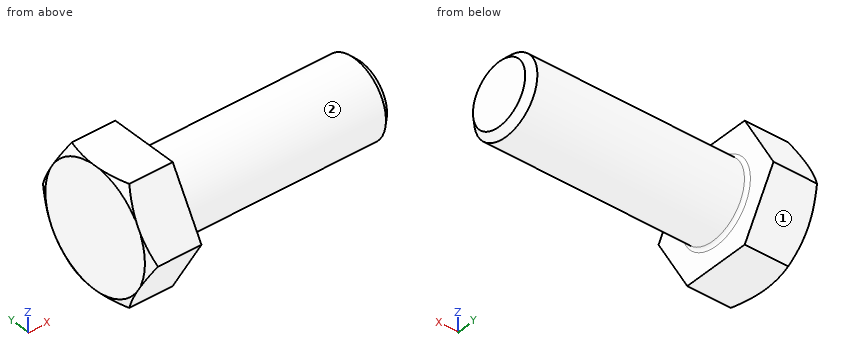
Autodesk Inventor part; units mm, degrees
ref_plane "Work Plane1" through (1.525, 0, 0) normal (0, 0, 1) x (1, 0, 0)
ref_plane "YZ Plane" through (0, 0, 0) normal (1, 0, 0) x (0, 1, 0)
ref_plane "XZ Plane" through (0, 0, 0) normal (0, 1, 0) x (-1, 0, 0)
sketch "Sketch1" plane through (0, 0, 0) normal (0, 0, 1) x (1, 0, 0)
  line L0 (0, 3.5) -> (20, 3.5)
  line L1 (20, 3.5) -> (20, 0)
  line L2 (20, 0) -> (0, 0)
  line L3 (-4, 0) -> (24, 0)
  line L4 (0, -0.7) -> (0, 4.2)
  line L5 (0, 3.5) -> (0, 0)
  dimension "d2" = 7
  dimension "d59" = 20
revolve "Body" add sketch "Sketch1" angle 360 about axis through (20, 0, 0) along (-1, 0, 0)
sketch "Sketch2" plane through (0, 0, 0) normal (-1, 0, 0) x (0, 0, 1)
  line L0 (0, 6.3509) -> (5.5, 3.1754)
  line L1 (5.5, 3.1754) -> (5.5, -3.1754)
  line L2 (5.5, -3.1754) -> (0, -6.3509)
  line L3 (0, -6.3509) -> (-5.5, -3.1754)
  line L4 (-5.5, -3.1754) -> (-5.5, 3.1754)
  line L5 (-5.5, 3.1754) -> (0, 6.3509)
  line L6 (-7.7, 0) -> (7.7, 0)
  line L7 (0, 8.8912) -> (0, -8.8912)
  point P0 (0, 0)
  point P1 (0, 0)
  dimension "d11" = 11
extrude "Head" add sketch "Sketch2" along normal blind 4.5
sketch "Sketch4" plane through (0, 0, 0) normal (0, 0, 1) x (1, 0, 0)
  line L0 (-3.8649, 6.6) -> (-4.5, 5.5)
  line L1 (-1.1, 0) -> (-0.234, 0)
  line L2 (-5.3532, 0) -> (0.6192, 0)
  line L3 (-4.5, 6.6) -> (-3.8649, 6.6)
  line L4 (-4.5, 5.5) -> (-4.5, 6.6)
  line L5 (0, 7.92) -> (0, -1.32)
  dimension "d65" = 11
  dimension "d67" = 30
  dimension "d68" = 13.2
  dimension "d69" = 4.5
revolve "Chamfer1" cut sketch "Sketch4" angle 360 about axis through (-1.1, 0, 0) along (1, 0, 0)
thread "Thread"
chamfer "Chamfer2" distance 0.6135 distance2 0.6136 1 edges at (20, -3.5, 0) measured on face at (20, 0.2032, -0.9043)
fillet "Fillet2" radius 0.3 1 edges at (0, -3.5, 0)
ref_plane "Work Plane1" through (1.525, 0, 0) normal (0, 0, 1) x (1, 0, 0)
equation "\"d2\" = GD"
equation "\"d59\" = NLG"
equation "\"d11\" = SW"
equation "\"d3\" = KOH"
equation "\"d71\" = RR"
equation "\"d15\" = GEL"
equation "\"d6\" = -0.5 * SPD + 0.5 * GD"
equation "\"d65\" = SW"
equation "\"d67\" = ANG1"
equation "\"d68\" = 1.2 * SW"
equation "\"d69\" = KOH"
equation "\"NLG\" = 20"
equation "\"GD\" = NND"
equation "\"BDM\" = NND"
equation "\"KOH\" = 4.5"
equation "\"GEL\" = 13"
equation "\"SW\" = 11"
equation "\"SW0\" = 11"
equation "\"SPD\" = NND - 1.2269 * PTC"
equation "\"SD2\" = NND"
equation "\"SD\" = 0"
equation "\"ANG1\" = 30deg"
equation "\"GAL\" = 0.61345 * PTC"
equation "\"GUL\" = 0.61345 * PTC"
equation "\"RR\" = 0.3"
equation "\"RR1\" = 0.1"
equation "\"GD1\" = THREADDIA - 1.2269 * PTC"
equation "\"THREADDIA\" = 7"
equation "\"TOA\" = 30deg"
equation "\"FAWI\" = 60deg"
equation "\"PTC\" = 1"
equation "\"NND\" = 7"
equation "\"E0\" = 1.155 * SW"
properties part number "CSN 02 1201 - M7 x 20" material "Steel, Mild"
Geometry: final body of the model. Coordinates: model frame, mm. Face numbers are marked on the shaded views. A direction names the side the tool comes from. Give positions to 0.01 mm unless a question says otherwise; leave off trailing zeros. Order: outer loops, then holes, each group sorted by start corner. A loop starts at its lowest first (then second) coordinate and runs counter-clockwise, first axis right, second up. Notation, with made-up numbers: (67.5, 69) -> (95.5, 69) arc R11 ccw to (95.5, 85) -> close; hole circle Ø6 at (-34, 7.25). An arc over 180 degrees is marked (long way). Put each result on its own line as item: value.
Q1. Section A-A, the plane x = 13.25. Return loops of the section in (y, z), then the cut area to 3 significant figures.
Here are the results:
outline: circle Ø7 at (0, 0)
area: 38.5 mm^2
Q2. Material intervals for L1, parallel to X at y = -2.5, z = -4.75; L2, parallel to Y at x = 5.25, z = -3; L3, parallel to X at y = -3, z = -1.5, sorted ascending.
Here are the results:
L1: x = -4.5 to 0
L2: y = -1.8 to 1.8
L3: x = -4.5 to 19.53
Q3. Pin query (flat end, axial travel): pin 1 (3 mm diameter, centred on x = 13.5, y = -2.5, fed in from +Z); pin 2 (1 mm diameter, centred on y = -3, z = -2.5, fed in from +X); pin 3 (4 mm diameter, centred on x = 8.5, y = 3.5, fed in from +Z). Return the tip coordinate at first contact, or that it passes through.
Here are the results:
pin 1: stops at z = 3.35
pin 2: stops at x = 19.48
pin 3: stops at z = 3.16
Q4. Reachability of the marked faces 1 and 2 from +Z, -Z, +X, -X, +Y, -Y: full face, straight path, thin tool, end or side. Return the list, or none.
Here are the results:
face 1: -Z, +X, -X, +Y
face 2: +X
